Build history of the part. All positions in model axes, mm. A direction names the side the tool comes from. Give positions to 0.01 mm unless a question says otherwise; leave off trailing zeros. Loops run counter-clockwise (first coordinate to the right, second up) from the corner with the lowest first, then second, coordinate; pieces in that order, holes last. Notation, with made-up numbers: (64, 66) - (102, 66) arc R9 ccw to (102, 71) - close; hole circle Ø6 at (21, 21). An arc over 180 degrees is marked (long way). Return JSON: item names as keys, results as strings. Group by question number.
1) Drill centre lines: probe 1 along X at (y, z) = (-312.5, 1); probe 2 along Y at (x, z) = (11.5, -13). Where is each one in solid material? Low to high. Write a range as from..to.
2) 3-axis set-ups, long thin cutter, end or side, ignore diameter. For faces 1 (the face through (11, -406.4, -12)), 2 (the face through (0, 0, 0)): which of +Z, -Z, +X, -X, +Y, -Y reach the whole face in a straight line?
3) Slice it at B-B (y = 19). List the corners of the cut face in (x, z) (3 decimals).
4) Slice it at A-A (y = -128.5). List the corners of the cut face in (x, z) (1 decimal), and give its area (3 significant figures).
5) Drop flat-ended pins along their axis: pin 1 (4 mm diameter, centred on x = 9, y = -345.5, fed in from -Z); pin 2 (1 mm diameter, centred on y = -165.5, z = -4.5, fed in from +X); pin 3 (5 mm diameter, centred on x = -15, y = -246.5, fed in from +Z); pin 4 (12.5 mm diameter, centred on x = 7.5, z = -1, fed in from +Y). Give the stop position or say it passes through.
6) Mould opens along X. For faces 3 (the face through (0, 12.7, -4)), 4 (the face through (-14.274, -199.573, 0.628)) say: released by +X, released by -X, zero draft, split by the parting line, or undercut.
```python
from build123d import *

# Parameters (mm, degrees)
F0_R     = 20.6375
F0_R_2   = 14.2875
F1_DEPTH = 406.4
F2_R     = 20.6375
F3_DEPTH = 12.7
F4_W     = 6.35
F4_H     = 6.35
F5_DEPTH = 38.1
F7_DEPTH = 25.4
F8_SIZE  = 1.5875


with BuildPart() as f1:
    # F0 (on Front) → F1 (new body)
    with BuildSketch(Plane.XZ):
        Circle(F0_R)
        Circle(F0_R_2, mode=Mode.SUBTRACT)
    extrude(amount=F1_DEPTH)

    # F2 (on face) → F3 (join)
    with BuildSketch(Plane(origin=(0, 0, 0), x_dir=(-1, 0, 0), z_dir=(0, 1, 0))):
        Circle(F2_R)
    extrude(amount=F3_DEPTH)

    # F4 (on face) → F5 (join)
    with BuildSketch(Plane(origin=(0, 12.7, 0), x_dir=(-1, 0, 0), z_dir=(0, 1, 0))):
        Rectangle(F4_W, F4_H)
    extrude(amount=F5_DEPTH)

    # F6 (on Top) → F7 (cut)
    with BuildSketch(Plane.XY):
        with BuildLine():
            ThreePointArc((0, -394.49375), (-2.80633, -401.26883), (3.96875, -398.4625))
            ThreePointArc((3.96875, -398.4625), (2.80633, -395.65617), (0, -394.49375))
        make_face()
    extrude(amount=F7_DEPTH, mode=Mode.SUBTRACT)

    # F8
    f8_edges = [f1.edges().sort_by_distance(p)[0] for p in [
        (-14.2875, -406.4, 0),
    ]]
    chamfer(f8_edges, length=F8_SIZE)


solid = f1.part
```
Results:
{
 "1": {"probe 1": "-20.61..-14.25, 14.25..20.61", "probe 2": "-406.4..12.7"},
 "2": {"face 1": "+Z, -Z, +X, -X, -Y", "face 2": "-Y"},
 "3": {"outline": "(-3.175, -3.175) - (3.175, -3.175) - (3.175, 3.175) - (-3.175, 3.175) - close"},
 "4": {"outline": "circle Ø41.3 at (0, 0); hole circle Ø28.6 at (0, 0)", "area": "697 mm2"},
 "5": {"pin 1": "z = -19.41", "pin 2": "x = 20.25", "pin 3": "z = 16.42", "pin 4": "y = 50.8"},
 "6": {"face 3": "zero draft", "face 4": "undercut"}
}
